from build123d import *

# Parameters (mm, degrees)
CROQUIS1_R              = 1.5
SALIENTE_EXTRUIR1_DEPTH = 10
CROQUIS3_R              = 2.5
SALIENTE_EXTRUIR3_DEPTH = 3
CORTAR_EXTRUIR1_DEPTH   = 2.5
REDONDEO4_R             = 0.1
REDONDEO5_R             = 0.1


with BuildPart() as part:
    # Croquis1 → Saliente-Extruir1 (new body)
    with BuildSketch(Plane.XY):
        Circle(CROQUIS1_R)
    extrude(amount=SALIENTE_EXTRUIR1_DEPTH)

    # Croquis3 → Saliente-Extruir3 (add)
    with BuildSketch(Plane(origin=(0, 0, 0), x_dir=(-1, 0, 0), z_dir=(0, 0, -1))):
        Circle(CROQUIS3_R)
    extrude(amount=SALIENTE_EXTRUIR3_DEPTH)

    # Croquis4 → Cortar-Extruir1 (cut)
    with BuildSketch(Plane(origin=(0, 0, -3), x_dir=(-1, 0, 0), z_dir=(0, 0, -1))):
        Polygon((1.5, 0), (0.75, 1.299038106), (-0.75, 1.299038106), (-1.5, 0), (-0.75, -1.299038106), (0.75, -1.299038106), align=None)
    extrude(amount=-CORTAR_EXTRUIR1_DEPTH, mode=Mode.SUBTRACT)

    # Redondeo4
    redondeo4_edges = [part.edges().sort_by_distance(p)[0] for p in [
        (2.5, 0, -3),
    ]]
    fillet(redondeo4_edges, radius=REDONDEO4_R)

    # Redondeo5
    redondeo5_edges = [part.edges().sort_by_distance(p)[0] for p in [
        (2.5, 0, 0),
    ]]
    fillet(redondeo5_edges, radius=REDONDEO5_R)


solid = part.part
Work out the finished part from the listing and answer in its coordinate system (mm). A direction names the side the tool comes from. Give positions to 0.01 mm unless a question says otherwise; leave off trailing zeros. Order: outer loops, then holes, each group sorted by start corner. A loop starts at its lowest first (then second) coordinate and runs counter-clockwise, first axis right, second up. Notation, with made-up numbers: M -16,70.5 L -5,70.5 A13 cw -5,80.5 Z; hole C 67,-6.75 d11. An arc over 180 degrees is marked long. Return JSON: item names as keys, results as strings.
Q1. Find section A-A, the plane x = 0. Write down the section's boundary in (y, z).
Answer below:
{"outline": "M -2.5,-2.9 A0.1 ccw -2.4,-3 L -1.3,-3 L -1.3,-0.5 L 1.3,-0.5 L 1.3,-3 L 2.4,-3 A0.1 ccw 2.5,-2.9 L 2.5,-0.1 A0.1 ccw 2.4,0 L 1.5,0 L 1.5,10 L -1.5,10 L -1.5,0 L -2.4,0 A0.1 ccw -2.5,-0.1 Z"}
Q2. Which of the six approach directions +Z, -Z, +X, -X, +Y, -Y give full straight-line access (tool end or side, diameter ignored) to faces 1 (the face through (0, -2, 0)), 2 (the face through (1.13, -0.64, -1.77)), 3 (the face through (0, -2, -3))?
Answer below:
{"face 1": "+Z", "face 2": "-Z", "face 3": "-Z, +X, -X, +Y, -Y"}
Q3. Find section B-B, the plane z = 4. Write down the section's boundary in (x, y), and give its area (3 significant figures).
Answer below:
{"outline": "C 0,0 d3", "area": "7.07 mm^2"}
Q4. Find the intervals of material crossed by line 1 along Z through (x, y) = (1, 1.5); line 2 along Z through (x, y) = (-0.1, -1.15); line 3 along X through (y, z) = (-0.1, 0.25), in increasing order. Write a range as [from, to].
Answer below:
{"line 1": "z = [-3, 0]", "line 2": "z = [-0.5, 10]", "line 3": "x = [-1.5, 1.5]"}
Q5. The mould has two halves that part along X. Classify faces 4 (the face through (-1.5, 0.07, 4.93)), 5 (the face through (0, 1.299, -2)), 6 (the face through (0, 0, 10)): pulls with the +X half, pulls with the -X half, needs draft (parallel to the pull), parting line crosses it, or undercut.
Answer below:
{"face 4": "parting line crosses it", "face 5": "undercut", "face 6": "needs draft"}
Q6. Each of these flat-tipped pins is pushed along its axis until it touches: pin 1 (1.5 mm diameter, centred on x = -0.5, z = 7, fed in from +Y); pin 2 (2 mm diameter, centred on x = 2, z = 2.5, fed in from -Y); pin 3 (3 mm diameter, centred on x = 0, y = 0, fed in from -Z); pin 4 (1 mm diameter, centred on x = 1.5, y = -2, fed in from +Z). Where does it stop, or does it pass through?
Answer below:
{"pin 1": "stops at y = 1.5", "pin 2": "stops at y = -1.12", "pin 3": "stops at z = -3", "pin 4": "stops at z = 0"}
